from build123d import *

# Parameters (mm, degrees)
ESQUISSE1_W             = 196
ESQUISSE1_H             = 309
ESQUISSE1_R             = 1.75
ESQUISSE1_R_2           = 3
BOSS_EXTRU_1_DEPTH      = 3
ENL_V_MAT_EXTRU_1_REACH = 5
CONG_1_R                = 5
ENL_V_MAT_EXTRU_2_DEPTH = 4
CONG_2_R                = 5


with BuildPart() as part:
    # Esquisse1 → Boss.-Extru.1 (new body)
    with BuildSketch(Plane.XY):
        Rectangle(ESQUISSE1_W, ESQUISSE1_H)
        with Locations((-81.5, 121.5)):
            Circle(ESQUISSE1_R, mode=Mode.SUBTRACT)
        with Locations((81.5, 121.5)):
            Circle(ESQUISSE1_R, mode=Mode.SUBTRACT)
        with Locations((81.5, -121.5)):
            Circle(ESQUISSE1_R, mode=Mode.SUBTRACT)
        with Locations((-81.5, -121.5)):
            Circle(ESQUISSE1_R, mode=Mode.SUBTRACT)
        with Locations((64.75, 121.5)):
            Circle(ESQUISSE1_R_2, mode=Mode.SUBTRACT)
        with Locations((-64.75, 121.5)):
            Circle(ESQUISSE1_R_2, mode=Mode.SUBTRACT)
        with Locations((-64.75, -121.5)):
            Circle(ESQUISSE1_R_2, mode=Mode.SUBTRACT)
        with Locations((64.75, -121.5)):
            Circle(ESQUISSE1_R_2, mode=Mode.SUBTRACT)
    extrude(amount=BOSS_EXTRU_1_DEPTH)

    # Esquisse2 → Enlèv. mat.-Extru.1 (cut, up to next)
    with BuildSketch(Plane.XY.offset(3), mode=Mode.PRIVATE) as enl_v_mat_extru_1_sk1:
        with BuildLine():
            Line((-15, -154.5), (-15, -115))
            ThreePointArc((-15, -115), (0, -100), (15, -115))
            Line((15, -115), (15, -154.5))
            ThreePointArc((15, -154.5), (0, -169.5), (-15, -154.5))
        make_face()
    enl_v_mat_extru_1_tool1 = extrude(enl_v_mat_extru_1_sk1.sketch, amount=-ENL_V_MAT_EXTRU_1_REACH, mode=Mode.PRIVATE) & part.part
    add(enl_v_mat_extru_1_tool1.solids().sort_by_distance((0, -134.75, 3))[0], mode=Mode.SUBTRACT)

    # Congé1
    cong_1_edges = [part.edges().sort_by_distance(p)[0] for p in [
        (-15, -154.5, 1.5),
        (15, -154.5, 1.5),
    ]]
    fillet(cong_1_edges, radius=CONG_1_R)

    # Esquisse3 → Enlèv. mat.-Extru.2 (cut, through all)
    with BuildSketch(Plane.XY.offset(3)):
        Polygon((-53, -28.5), (14, -28.5), (14, -6.5), (47, -6.5), (47, -87.5), (14, -87.5), (14, -45.5), (-53, -45.5), align=None)
    extrude(amount=-ENL_V_MAT_EXTRU_2_DEPTH, mode=Mode.SUBTRACT)

    # Congé2
    cong_2_edges = [part.edges().sort_by_distance(p)[0] for p in [
        (-53, -45.5, 1.5),
        (-53, -28.5, 1.5),
        (14, -6.5, 1.5),
        (47, -6.5, 1.5),
        (47, -87.5, 1.5),
        (14, -87.5, 1.5),
    ]]
    fillet(cong_2_edges, radius=CONG_2_R)


solid = part.part
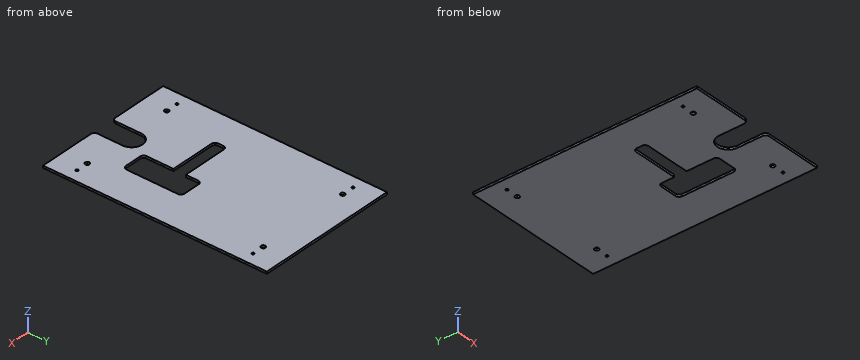
Can you work these out from the model? Positions are in its coordinate system, mm. Give positions to 0.01 mm unless a question says otherwise; leave off trailing zeros. Loops run counter-clockwise (first coordinate to the right, second up) from the corner with the lowest first, then second, coordinate; pieces in that order, holes last. Notation, with made-up numbers: (0, 76.5) - (13, 76.5) arc R12 cw to (13, 94.5) - close; hole circle Ø6 at (33.5, -38). An arc over 180 degrees is marked (long way). Answer as a JSON object with one key per item and string values.
Q1. If I drill on L1, parallel to Y at x = -64.75, z = 0.75; L2, parallel to Y at x = -81.5, z = 1.55; L3, parallel to Y at x = 25.5, z = 1.9, over which ranges is the centre line in solid material (lowest first)?
Geometry says:
{"L1": "-154.5 to -124.5, -118.5 to 118.5, 124.5 to 154.5", "L2": "-154.5 to -123.25, -119.75 to 119.75, 123.25 to 154.5", "L3": "-154.5 to -87.5, -6.5 to 154.5"}
Q2. Imagine slicing it at C-C on x = -28.5. Write out the boundary of the cut face in (y, z), plus the area to 3 significant figures.
Geometry says:
{"outline": "(-154.5, 0) - (-45.5, 0) - (-45.5, 3) - (-154.5, 3) - close; (-28.5, 0) - (154.5, 0) - (154.5, 3) - (-28.5, 3) - close", "area": "876 mm²"}
Q3. Imagine slicing it at D-D on x = 25.5. Write out the boundary of the cut face in (y, z).
Geometry says:
{"outline": "(-154.5, 0) - (-87.5, 0) - (-87.5, 3) - (-154.5, 3) - close; (-6.5, 0) - (154.5, 0) - (154.5, 3) - (-6.5, 3) - close"}
Q4. Imagine slicing it at A-A on z = 1. Give the number of separate pieces and of enclosed holes in the cut face, plus the area to 3 significant figures.
Geometry says:
{"separate pieces": "1", "enclosed holes": "9", "area": "55,100 mm²"}
Q5. Will these pins go through, and if not, where does the flat tip stop? P1, Ø8, axis at x = 64.75, y = -121.5, coming from the +Z side; P2, Ø0.9, axis at x = -7, z = 1.5, coming from the -Y side; P3, Ø5, axis at x = 64.75, y = 121.5, coming from the -Z side.
Geometry says:
{"P1": "z = 3", "P2": "y = -101.98", "P3": "through"}
Q6. Imagine slicing it at B-B on x = 64.75. Write out the boundary of the cut face in (y, z), plus the area to 3 significant figures.
Geometry says:
{"outline": "(-154.5, 0) - (-124.5, 0) - (-124.5, 3) - (-154.5, 3) - close; (-118.5, 0) - (118.5, 0) - (118.5, 3) - (-118.5, 3) - close; (124.5, 0) - (154.5, 0) - (154.5, 3) - (124.5, 3) - close", "area": "891 mm²"}
